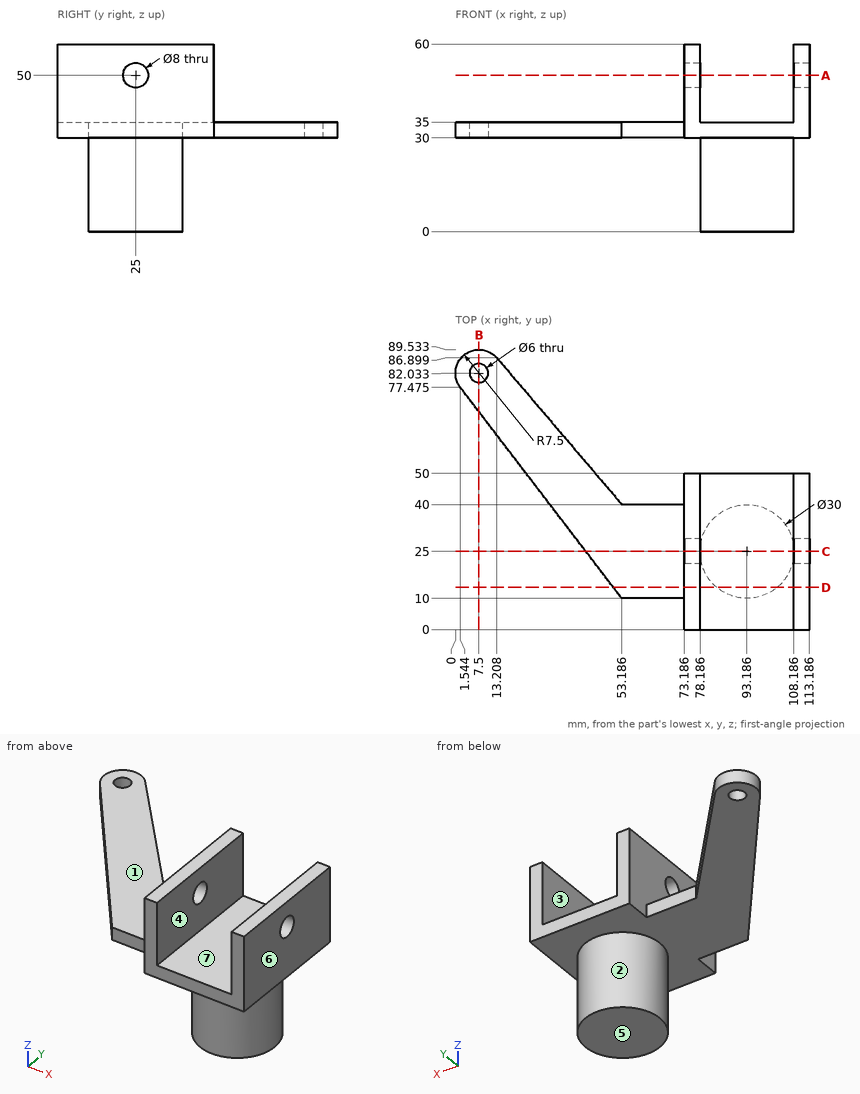
For this review, use the dimensioned drawing (mm, ordinates from the lowest corner) and the shaded views. A direction names the side the tool comes from. Give positions to 0.01 mm unless a question says otherwise; leave off trailing zeros. Order: outer loops, then holes, each group sorted by start corner. A loop starts at its lowest first (then second) coordinate and runs counter-clockwise, first axis right, second up. Notation, with made-up numbers: M 64.5,-19 L 71.5,-19 A27 cw 71.5,14 Z; hole C 21,18 d8. An arc over 180 degrees is marked long. Use one line per item in the form item = value. Start each with the question number.
Item 1: We need section B-B on x = 7.5. Give the boundary of the cut face in (y, z), plus the area to 3 significant figures.
Item 2: The part is to be moulded in two halves that separate along X. For the marked faces 4, 5, 6 and 7, say which applies: pulls with the +X half, pulls with the -X half, needs draft (parallel to the pull), parting line crosses it, or undercut.
Item 3: We need section A-A on z = 50. Give the boundary of the cut face in (x, y).
Item 4: Insertion check: pin 1 Ø13 at (y, z) = (25, 50) entering from +X; pin 2 Ø8 at (x, y) = (7.5, 82.03) entering from +Z; pin 3 Ø1.5 at (y, z) = (21, 20.5) entering from -X; pin 4 Ø1.5 at (x, z) = (59.5, 32.5) entering from -Y. Each pin has a flat end and moves straight along its axis. Give the tip position at first contact, or say it passes through.
Item 5: We need section C-C on y = 25. Give the boundary of the cut face in (x, z) (1 decimal).
Item 6: For the marked faces 1, 2 and 3, list the 3-axis set-ups (+Z, -Z, +X, -X, +Y, -Y) from which the entire face can be reached by the end or side of a thin tool; tool diameter is ignored.
Item 7: We need section D-D on y = 13.5. Give the boundary of the cut face in (x, z) (1 decimal).
Item 8: To check wall thickness, follow line 1 along X through (y, z) = (47, 55); line 2 along Y through (x, z) = (76, 50); line 3 along Z through (x, y) = (44.5, 35). State the ranges of each line that lie inside material, in increasing order. Write a range as from..to.
Completed:
q1.outline = M 69.69,30 L 79.03,30 L 79.03,35 L 69.69,35 Z; M 85.03,30 L 89.53,30 L 89.53,35 L 85.03,35 Z
q1.area = 69.2 mm²
q2.face_4 = undercut
q2.face_5 = needs draft
q2.face_6 = pulls with the +X half
q2.face_7 = undercut
q3.outline = M 73.19,0 L 78.19,0 L 78.19,21 L 73.19,21 Z; M 73.19,29 L 78.19,29 L 78.19,50 L 73.19,50 Z; M 108.19,0 L 113.19,0 L 113.19,21 L 108.19,21 Z; M 108.19,29 L 113.19,29 L 113.19,50 L 108.19,50 Z
q4.pin_1 = 113.19
q4.pin_2 = 35
q4.pin_3 = 78.54
q4.pin_4 = 10
q5.outline = M 41.7,30 L 78.2,30 L 78.2,0 L 108.2,0 L 108.2,30 L 113.2,30 L 113.2,46 L 108.2,46 L 108.2,35 L 78.2,35 L 78.2,46 L 73.2,46 L 73.2,35 L 41.7,35 Z; M 73.2,54 L 78.2,54 L 78.2,60 L 73.2,60 Z; M 108.2,54 L 113.2,54 L 113.2,60 L 108.2,60 Z
q6.face_1 = +Z, -X, +Y, -Y
q6.face_2 = -Z
q6.face_3 = +Z, +Y, -Y
q7.outline = M 50.5,30 L 83.6,30 L 83.6,0 L 102.8,0 L 102.8,30 L 113.2,30 L 113.2,60 L 108.2,60 L 108.2,35 L 78.2,35 L 78.2,60 L 73.2,60 L 73.2,35 L 50.5,35 Z
q8.line_1 = 73.19..78.19, 108.19..113.19
q8.line_2 = 0..21, 29..50
q8.line_3 = 30..35
